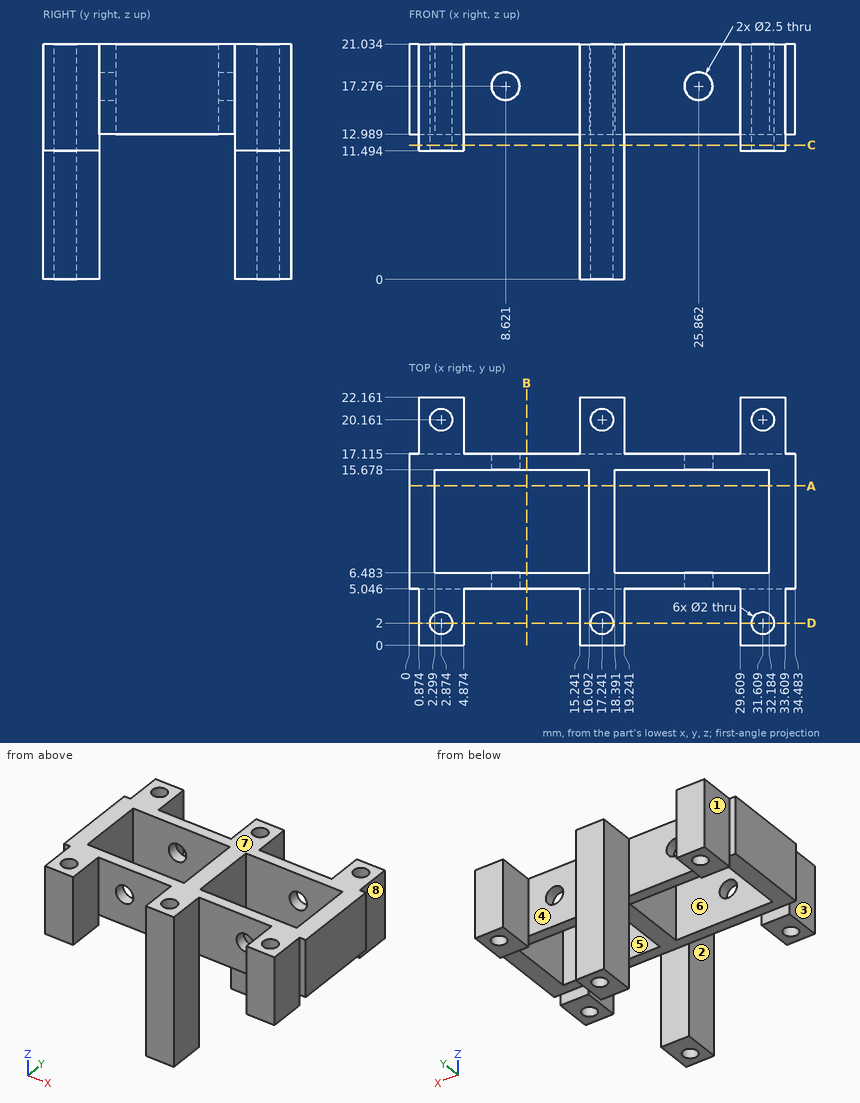
Input: dimensioned drawing with shaded views. Units: mm. Origin: part minimum x, y, z. A direction names the side the tool comes from. Round coordinates to 2 decimals unless told otherwise and drop trailing zeros. Order: outer loops, then holes, each group sorted by start corner. A loop starts at its lowest first (then second) coordinate and runs counter-clockwise, first axis right, second up.
1. Mould query, pull axis X, two halves, no side actions, for the marked faces 6, 7 and 8. Classes: released by +X, released by -X, zero draft, split by the parting line, or undercut.
The answers:
face 6: undercut
face 7: zero draft
face 8: released by +X
2. Set-up query: the marked faces 1, 2, 3, 4 and 5. Return all of +Z, -Z, +X, -X, +Y, -Y with unobstructed straight access to the full face (end or side cutting, diameter ignored); none if empty.
The answers:
face 1: +Z, -Z, -X, +Y
face 2: +Z, -Z, -Y
face 3: +Z, -Z, -X, -Y
face 4: +Z, -Z, +Y
face 5: +Z, -Z
3. Material intervals for line 1 (X direction, y = 3.5, z = 20.25); line 2 (X direction, y = 13.5, z = 15); line 3 (X direction, y = 2.5, z = 13.5) (1 decimal), sorted ascending.
The answers:
line 1: x = 0.87 to 4.87, 15.24 to 19.24, 29.61 to 33.61
line 2: x = 0 to 2.3, 16.09 to 18.39, 32.18 to 34.48
line 3: x = 0.9 to 2, 3.7 to 4.9, 15.2 to 16.4, 18.1 to 19.2, 29.6 to 30.7, 32.5 to 33.6
4. Cut plane B-B, the plane x = 10.5. Output: boundary loops of the cut face in (y, z) (1 decimal).
The answers:
outline: (5, 13) - (6.5, 13) - (6.5, 21) - (5, 21) - close; (15.7, 13) - (17.1, 13) - (17.1, 21) - (15.7, 21) - close
5. Cut plane D-D, the plane y = 2. Output: boundary loops of the cut face in (x, z) (1 decimal).
The answers:
outline: (0.9, 11.5) - (1.9, 11.5) - (1.9, 21) - (0.9, 21) - close; (3.9, 11.5) - (4.9, 11.5) - (4.9, 21) - (3.9, 21) - close; (15.2, 0) - (16.2, 0) - (16.2, 21) - (15.2, 21) - close; (18.2, 0) - (19.2, 0) - (19.2, 21) - (18.2, 21) - close; (29.6, 11.5) - (30.6, 11.5) - (30.6, 21) - (29.6, 21) - close; (32.6, 11.5) - (33.6, 11.5) - (33.6, 21) - (32.6, 21) - close
6. Cut plane A-A, the plane y = 14.25. Output: boundary loops of the cut face in (x, z) (1 decimal).
The answers:
outline: (0, 13) - (2.3, 13) - (2.3, 21) - (0, 21) - close; (16.1, 13) - (18.4, 13) - (18.4, 21) - (16.1, 21) - close; (32.2, 13) - (34.5, 13) - (34.5, 21) - (32.2, 21) - close
7. Cut plane C-C, the plane z = 12. State how many separate pieces and enclosed holes the cut face has, then the cut area to 3 significant figures.
The answers:
separate pieces: 6
enclosed holes: 6
area: 102 mm2
8. Pin query (flat end, axial travel): P1, Ø1.8, axis at x = 31.61, y = 2, coming from the +Z side; P2, Ø2.5, axis at x = 17.24, y = 20.16, coming from the +Z side (1 decimal); P3, Ø1.5, axis at y = 3, z = 14.5, coming from the -X side; P4, Ø2, axis at x = 31, y = 19.5, coming from the -Z side. Return the tip coordinate at first contact, or that it passes through.
The answers:
P1: passes through
P2: stops at z = 21
P3: stops at x = 0.87
P4: stops at z = 11.49
